Verification items for the finished model (mm, model axes). Face numbers are marked on the shaded views. A direction names the side the tool comes from. Round coordinates to 2 decimals unless told otherwise and drop trailing zeros. Loops run counter-clockwise (first coordinate to the right, second up) from the corner with the lowest first, then second, coordinate; pieces in that order, holes last. Notation, with made-up numbers: (49, 81) -> (107, 81) arc R33 ccw to (107, 111) -> close; hole circle Ø8 at (23.5, 13). An arc over 180 degrees is marked (long way). Write item = value, one per line.
```python
from build123d import *

# Parameters (mm, degrees)
PAD6703_DEPTH            = 63.5
FILLET540_R              = 6.35
FILLET541_R              = 3.175
SKETCH7626_R             = 2.38125
POCKET658_DEPTH          = 12.701
CHAMFER2378_SIZE         = 3.175
BODY6012_PLACEMENT_ANGLE = 180


with BuildPart() as part:
    # Sketch7640 → Pad6703 (new body, symmetric)
    with BuildSketch(Plane.XZ):
        Polygon((0, 0), (22.098, 0), (22.098, -9.398), (25.4, -9.398), (25.4, 3.302), (0, 3.302), align=None)
    extrude(amount=PAD6703_DEPTH, both=True)

    # Fillet540
    fillet540_edges = [part.edges().sort_by_distance(p)[0] for p in [
        (23.749, -63.5, -9.398),
        (23.749, 63.5, -9.398),
        (0, 63.5, 1.651),
        (0, -63.5, 1.651),
    ]]
    fillet(fillet540_edges, radius=FILLET540_R)

    # Fillet541
    fillet541_edges = [part.edges().sort_by_distance(p)[0] for p in [
        (25.4, 0, 3.302),
    ]]
    fillet(fillet541_edges, radius=FILLET541_R)

    # Sketch7626 (on ShapeBinder) → Pocket658 (cut, through all)
    with BuildSketch(Plane(origin=(0, 0, 3.302), x_dir=(-1, 0, 0), z_dir=(0, 0, 1))):
        with Locations((-7.9375, 53.975)):
            Circle(SKETCH7626_R)
        with Locations((-7.9375, -53.975)):
            Circle(SKETCH7626_R)
    extrude(amount=-POCKET658_DEPTH, mode=Mode.SUBTRACT)

    # Chamfer2378
    chamfer2378_edges = [part.edges().sort_by_distance(p)[0] for p in [
        (10.31875, 53.975, 3.302),
        (10.31875, -53.975, 3.302),
    ]]
    chamfer(chamfer2378_edges, length=CHAMFER2378_SIZE)


with BuildPart() as part_1:
    # Body6007 placement: moved
    add(part.part.moved(Location((4.7625, 0, 146.05))))


with BuildPart() as part_2:
    # Clone377 placement: moved
    add(part_1.part.moved(Location((0, -19.05, -142.875))))


with BuildPart() as part_3:
    # Body6012 placement: moved
    add(part_2.part.moved(Location((0, -19.05, -142.875))).rotate(Axis((0, -19.05, -142.875), (1, 0, 0)), BODY6012_PLACEMENT_ANGLE))


solid = part_3.part
```
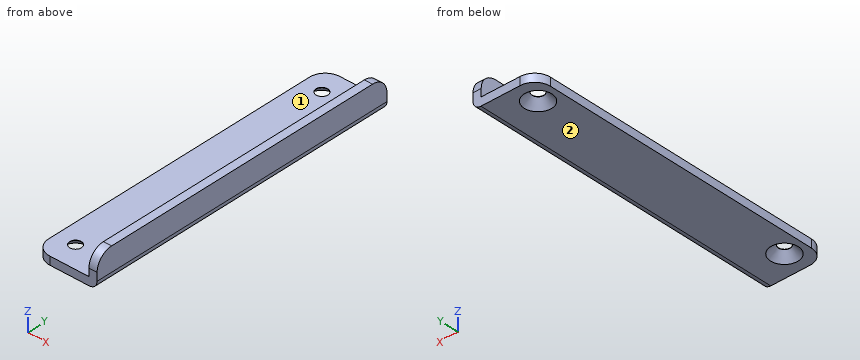
(1) Sectioned sample at C-C, the plane z = -145. Record the cut outline in (x, y), and give its area (3 significant figures).
Filled sheet:
outline = (26.86, -63.5) -> (30.16, -63.5) -> (30.16, 63.5) -> (26.86, 63.5) -> close
area = 419 mm2
(2) Material ranges on probe 1 along Y at (x, z) = (12.7, -146.1); probe 2 along Y at (x, z) = (12.25, -148.5); probe 3 along X at (y, z) = (20.5, -142.5), recorded low to high. Write a range as from..to.
Filled sheet:
probe_1 = -63.5..-56.36, -51.59..51.59, 56.36..63.5
probe_2 = -63.5..-58.66, -49.29..49.29, 58.66..63.5
probe_3 = 26.86..30.16
(3) Sectioned sample at D-D, the plane x = 21.25. Record the cut outline in (y, z).
Filled sheet:
outline = (-63.5, -149.35) -> (63.5, -149.35) -> (63.5, -146.05) -> (-63.5, -146.05) -> close
(4) Sectioned sample at A-A, the plane x = 12.7. Record the cut outline in (y, z), and give its area (3 significant figures).
Filled sheet:
outline = (-63.5, -149.35) -> (-59.53, -149.35) -> (-56.36, -146.18) -> (-56.36, -146.05) -> (-63.5, -146.05) -> close; (-51.59, -146.18) -> (-48.42, -149.35) -> (48.42, -149.35) -> (51.59, -146.18) -> (51.59, -146.05) -> (-51.59, -146.05) -> close; (56.36, -146.18) -> (59.53, -149.35) -> (63.5, -149.35) -> (63.5, -146.05) -> (56.36, -146.05) -> close
area = 368 mm2
(5) Set-up check for the marked faces 1 and 2: record each of +Z, -Z, +X, -X, +Y, -Y from which the full face is reachable in a straight line by a thin tool's end or side.
Filled sheet:
face_1 = +Z, -X, +Y, -Y
face_2 = -Z, +X, -X, +Y, -Y
(6) Go/stop test with flat-tipped pins: pin 1 Ø1 at (x, z) = (9.5, -146.5) entering from +Y; pin 2 Ø7.5 at (x, y) = (12.7, -53.975) entering from +Z; pin 3 Ø3 at (x, y) = (12.7, 53.975) entering from +Z; pin 4 Ø6 at (y, z) = (-43.5, -138.5) entering from -X. Record where each tip stops, or that it passes through.
Filled sheet:
pin_1 = 63.4
pin_2 = -146.05
pin_3 = through
pin_4 = 26.86
